Geometry check sheet. Reference: the model listing, model coordinates, mm. Face numbers are marked on the shaded views. A direction names the side the tool comes from. Round coordinates to 2 decimals unless told otherwise and drop trailing zeros. Order: outer loops, then holes, each group sorted by start corner. A loop starts at its lowest first (then second) coordinate and runs counter-clockwise, first axis right, second up. Notation, with made-up numbers: (68.25, 62) - (109.25, 62) arc R16 ccw to (109.25, 69) - close; hole circle Ø2 at (28, 60.5). An arc over 180 degrees is marked (long way). Return JSON: item names as keys, results as strings. Group by question number.
Q1. Gauge pin test, flat ends, axial feed: pin 1 Ø14 at (y, z) = (17.5, -1.5) entering from -X; pin 2 Ø5 at (y, z) = (11, -2.5) entering from +X; pin 3 Ø9.5 at (x, z) = (22.5, 0) entering from +Y. Record the tip position at first contact, or that the pin passes through.
Q2. Sectioned sample at B-B, the plane z = 0. Give the number of separate pieces and of enclosed holes in the cut face, then the cut area to 3 significant figures.
Q3. Sectioned sample at D-D, the plane x = 13. Record the cut outline in (y, z), then the cut area to 3 significant figures.
Q4. Tool access check on the marked faces 1, 2 and 3. Record the directions out of +Z, -Z, +X, -X, +Y, -Y that give a thin tool (end or side, any length) a straight path to the whole face; none if there is none.
Q5. Sectioned sample at A-A, the plane x = -22.5. Record the cut outline in (y, z).
Q6. Sectioned sample at C-C, the plane y = 20.25. Record the cut outline in (x, z), then the cut area to 3 significant figures.
Q7. Material ranges on line 1 along X through (y, z) = (3.5, 0); line 2 along X through (y, z) = (18, -9.25); line 3 along Z through (x, y) = (6, 21.75), recorded low to high.
Q8. Draft check along Z on the marked faces 4, 5, 6 and 7. Enter one of: pulls with the +Z half, pulls with the -Z half, needs draft (parallel to the pull), parting line crosses it, or undercut.
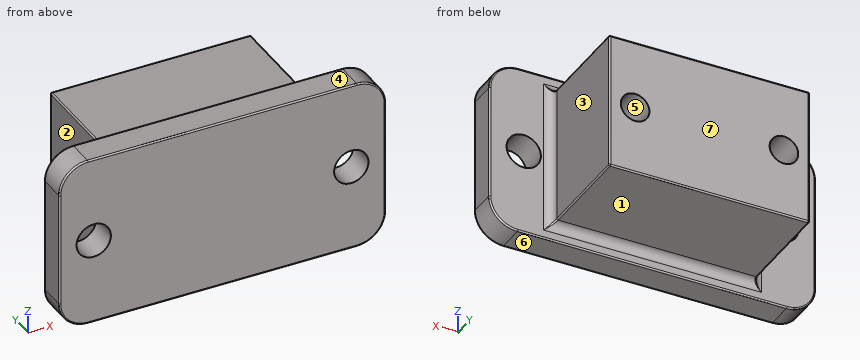
```python
from build123d import *

# Parameters (mm, degrees)
SKETCH1_R           = 3
BOSS_EXTRUDE1_DEPTH = 5
SKETCH2_W           = 35
SKETCH2_H           = 19
BOSS_EXTRUDE2_DEPTH = 12
SKETCH3_R           = 2.5
CUT_EXTRUDE1_DEPTH  = 13
FILLET1_R           = 1.5
FILLET2_R           = 0.25
FILLET3_R           = 0.25


with BuildPart() as part:
    # Sketch1 → Boss-Extrude1 (new body)
    with BuildSketch(Plane(origin=(0, 0, 0), x_dir=(1, 0, 0), z_dir=(0, 1, 0))):
        with BuildLine():
            Line((23.5, -15), (-23.5, -15))
            ThreePointArc((-23.5, -15), (-27.035533906, -13.535533906), (-28.5, -10))
            Line((-28.5, -10), (-28.5, 10))
            ThreePointArc((-28.5, 10), (-27.035533906, 13.535533906), (-23.5, 15))
            Line((-23.5, 15), (23.5, 15))
            ThreePointArc((23.5, 15), (27.035533906, 13.535533906), (28.5, 10))
            Line((28.5, 10), (28.5, -10))
            ThreePointArc((28.5, -10), (27.035533906, -13.535533906), (23.5, -15))
        make_face()
        with Locations(Location((-22.5, 0, 0), (0, 0, 270))):
            Circle(SKETCH1_R, mode=Mode.SUBTRACT)
        with Locations(Location((22.5, 0, 0), (0, 0, 270))):
            Circle(SKETCH1_R, mode=Mode.SUBTRACT)
    extrude(amount=BOSS_EXTRUDE1_DEPTH)

    # Sketch2 → Boss-Extrude2 (add, symmetric)
    with BuildSketch(Plane.XY):
        with Locations((0, 14.5)):
            Rectangle(SKETCH2_W, SKETCH2_H)
    extrude(amount=BOSS_EXTRUDE2_DEPTH, both=True)

    # Sketch3 → Cut-Extrude1 (cut)
    with BuildSketch(Plane(origin=(0, 24, 0), x_dir=(1, 0, 0), z_dir=(0, 1, 0))):
        with Locations(Location((-13, 0, 0), (0, 0, 180))):
            Circle(SKETCH3_R)
        with Locations(Location((13, 0, 0), (0, 0, 180))):
            Circle(SKETCH3_R)
    extrude(amount=-CUT_EXTRUDE1_DEPTH, mode=Mode.SUBTRACT)

    # Fillet1
    fillet1_edges = [part.edges().sort_by_distance(p)[0] for p in [
        (0, 5, -12),
        (-17.5, 5, 0),
        (17.5, 5, 0),
        (0, 5, 12),
    ]]
    fillet(fillet1_edges, radius=FILLET1_R)

    # Fillet2
    fillet2_edges = [part.edges().sort_by_distance(p)[0] for p in [
        (28.5, 0, 0),
        (27.035533906, 0, 13.535533906),
        (0, 0, 15),
        (-27.035533906, 0, 13.535533906),
        (27.035533906, 5, 13.535533906),
        (28.5, 5, 0),
        (27.035533906, 5, -13.535533906),
        (0, 5, -15),
        (-27.035533906, 5, -13.535533906),
        (-28.5, 5, 0),
        (-27.035533906, 5, 13.535533906),
        (-28.5, 0, 0),
        (0, 5, 15),
        (-27.035533906, 0, -13.535533906),
        (0, 0, -15),
        (27.035533906, 0, -13.535533906),
    ]]
    fillet(fillet2_edges, radius=FILLET2_R)

    # Fillet3
    fillet3_edges = [part.edges().sort_by_distance(p)[0] for p in [
        (-17.5, 15.25, -12),
        (-17.5, 24, 0),
        (0, 24, -12),
        (17.5, 24, 0),
        (-17.5, 15.25, 12),
        (0, 24, 12),
        (17.5, 15.25, -12),
        (17.5, 15.25, 12),
        (18.030926639, 5.355055975, 12.530926639),
        (18.030926639, 5.355055975, -12.530926639),
        (-18.030926639, 5.355055975, 12.530926639),
        (-18.030926639, 5.355055975, -12.530926639),
    ]]
    fillet(fillet3_edges, radius=FILLET3_R)


solid = part.part
```
Reply:
{
 "1": {"pin 1": "x = -17.5", "pin 2": "x = 17.5", "pin 3": "y = 5.67"},
 "2": {"separate pieces": "3", "enclosed holes": "0", "area": "761 mm^2"},
 "3": {"outline": "(0, -14.75) arc R0.25 ccw to (0.25, -15) - (4.75, -15) arc R0.25 ccw to (5, -14.75) - (5, -13.5) arc R1.5 cw to (6.5, -12) - (23.75, -12) arc R0.25 ccw to (24, -11.75) - (24, -2.5) - (11, -2.5) - (11, 2.5) - (24, 2.5) - (24, 11.75) arc R0.25 ccw to (23.75, 12) - (6.5, 12) arc R1.5 cw to (5, 13.5) - (5, 14.75) arc R0.25 ccw to (4.75, 15) - (0.25, 15) arc R0.25 ccw to (0, 14.75) - close", "area": "542 mm^2"},
 "4": {"face 1": "-Z, +X, -X, +Y", "face 2": "+Z, -Z, -X, +Y", "face 3": "+Z, -Z, +X, +Y"},
 "5": {"outline": "(0, -14.75) arc R0.25 ccw to (0.25, -15) - (4.75, -15) arc R0.25 ccw to (5, -14.75) - (5, -3) - (0, -3) - close; (0, 3) - (5, 3) - (5, 14.75) arc R0.25 ccw to (4.75, 15) - (0.25, 15) arc R0.25 ccw to (0, 14.75) - close"},
 "6": {"outline": "(-17.5, -11.75) arc R0.25 ccw to (-17.25, -12) - (17.25, -12) arc R0.25 ccw to (17.5, -11.75) - (17.5, 11.75) arc R0.25 ccw to (17.25, 12) - (-17.25, 12) arc R0.25 ccw to (-17.5, 11.75) - close; hole circle Ø5 at (-13, 0); hole circle Ø5 at (13, 0)", "area": "801 mm^2"},
 "7": {"line 1": "-28.5 to -25.5, -19.5 to 19.5, 25.5 to 28.5", "line 2": "-17.5 to 17.5", "line 3": "-12 to 12"},
 "8": {"face 4": "pulls with the +Z half", "face 5": "undercut", "face 6": "pulls with the -Z half", "face 7": "needs draft"}
}
